Source: CAD feature listing. Evaluate the final solid. Frame: model axes, mm. A direction names the side the tool comes from. Round coordinates to 2 decimals unless told otherwise and drop trailing zeros. Loops run counter-clockwise (first coordinate to the right, second up) from the corner with the lowest first, then second, coordinate; pieces in that order, holes last.
Item 1: Section query C-C on y = 25. Return loops of the section in (x, z), then the cut area to 3 significant figures.
Item 2: Section query B-B on z = 16. Return loops of the section in (x, y), then the cut area to 3 significant figures.
Item 3: Section query D-D on z = 8. Return loops of the section in (x, y).
Item 4: Pull-direction query (Z, two-part tool) for faces 1 (the cylindrical face through (-47, 6.6, -6.5)), 2 (the flat face through (-1, 9, 28.5)), 3 (the flat face through (-1, 0, 0)), 4 (the cylindrical face through (-50.845, 6.591, 11.091)); classes: released by +Z, released by -Z, zero draft, split by the parting line, or undercut.
Item 5: Section query A-A on x = -44.5. Return loops of the section in (y, z), then the cut area to 3 significant figures.
Item 6: Access query for faces 5 (the flat face through (60.5, 9, 0)), 6 (the flat face through (46.811, 23.778, -10.444)), 7 (the flat face through (-25.5, 24, 0)), 8 (the flat face through (4, 35, 6.5)). Directions: +Z, -Z, +X, -X, +Y, -Y. A direction counts if a zero-diameter tool reaches every point of the face in a straight line with its end or side. Return the directions, or none.
Item 7: First-contact query: P1, Ø5, axis at x = -21.5, z = 5.5, coming from the +Y side; P2, Ø2, axis at x = 24.5, y = 25, coming from the +Z side; P3, Ø1.5, axis at x = -22, z = 11, coming from the +Y side; P4, Ø10.5, axis at x = -44.5, z = 12.5, coming from the -Y side (3 decimals). Flat tips, straight axial feed; report the tip coordinate or a pass-through.
Item 8: Ray query, L1, parallel to Z at x = -44, y = 10; L2, parallel to X at y = 2.5, z = -12.5; L3, parallel to Z at x = 3, y = 26. Return the intervals inside material, ascending.
```python
from build123d import *

# Parameters (mm, degrees)
SKETCH1_W           = 121
SKETCH1_H           = 57
BOSS_EXTRUDE1_DEPTH = 13
SKETCH3_W           = 86
SKETCH3_H           = 41
BOSS_EXTRUDE2_DEPTH = 57
CUT_EXTRUDE1_DEPTH  = 41
BOSS_EXTRUDE3_START = -57
BOSS_EXTRUDE3_DEPTH = 57
CUT_EXTRUDE3_DEPTH  = 100.122399083
CUT_EXTRUDE4_REACH  = 101.122
CUT_EXTRUDE5_REACH  = 101.122
SKETCH10_R          = 6.5
CUT_EXTRUDE6_DEPTH  = 79.444247718


with BuildPart() as part:
    # Sketch1 → Boss-Extrude1 (new body)
    with BuildSketch(Plane(origin=(0, 0, 0), x_dir=(1, 0, 0), z_dir=(0, 1, 0))):
        Rectangle(SKETCH1_W, SKETCH1_H)
    extrude(amount=BOSS_EXTRUDE1_DEPTH)

    # Sketch3 → Boss-Extrude2 (add)
    with BuildSketch(Plane.XY.offset(28.5)):
        with Locations((17.5, 33.5)):
            Rectangle(SKETCH3_W, SKETCH3_H)
    extrude(amount=-BOSS_EXTRUDE2_DEPTH)

    # Sketch5 → Cut-Extrude1 (cut)
    with BuildSketch(Plane(origin=(0, 54, 0), x_dir=(1, 0, 0), z_dir=(0, 1, 0))):
        Polygon((-25.5, -6.5), (33.5, -6.5), (60.5, -14.5), (60.5, -28.5), (-25.5, -28.5), align=None)
        Polygon((33.5, 6.5), (60.5, 14.5), (60.5, 28.5), (-25.5, 28.5), (-25.5, 6.5), align=None)
    extrude(amount=-CUT_EXTRUDE1_DEPTH, mode=Mode.SUBTRACT)

    # Sketch6 → Boss-Extrude3 (add)
    with BuildSketch(Plane.XY.offset(28.5).offset(BOSS_EXTRUDE3_START)):
        Polygon((-25.5, 32), (60.5, 8.956369451), (-25.5, 13), align=None)
    extrude(amount=BOSS_EXTRUDE3_DEPTH)

    # Sketch7 → Cut-Extrude3 (cut, through all)
    with BuildSketch(Plane.XY.offset(28.5)):
        Polygon((-25.5, 54), (33.536835762, 38.181127534), (60.5, 22.613937403), (60.5, 54), align=None)
    extrude(amount=-CUT_EXTRUDE3_DEPTH, mode=Mode.SUBTRACT)

    # Cut-Extrude4: up to this face of the body (flat: up to its plane)
    cut_extrude4_end = Plane(part.part.faces().sort_by_distance((45.301820021, 22.632080787, 9.996835562))[0])
    # Sketch8 → Cut-Extrude4 (cut, up to the picked face)
    with BuildSketch(Plane.XY.offset(28.5), mode=Mode.PRIVATE) as cut_extrude4_sk1:
        Polygon((45.408965344, 13), (60.5, 13), (60.5, 8.956369451), align=None)
    cut_extrude4_tool1 = split(extrude(cut_extrude4_sk1.sketch, amount=-CUT_EXTRUDE4_REACH, mode=Mode.PRIVATE), bisect_by=cut_extrude4_end, keep=Keep.BOTH, mode=Mode.PRIVATE)
    add(cut_extrude4_tool1.solids().sort_by(Axis((55.469655, 11.652123, 28.5), (0, 0, -1)))[0], mode=Mode.SUBTRACT)

    # Cut-Extrude5: up to this face of the body (flat: up to its plane)
    cut_extrude5_end = Plane(part.part.faces().sort_by_distance((45.301820021, 22.632080787, -9.996835562))[0])
    # Sketch9 → Cut-Extrude5 (cut, up to the picked face)
    with BuildSketch(Plane(origin=(0, 0, -28.5), x_dir=(-1, 0, 0), z_dir=(0, 0, -1)), mode=Mode.PRIVATE) as cut_extrude5_sk1:
        Polygon((-45.408965344, 13), (-60.5, 13), (-60.5, 8.956369451), align=None)
    cut_extrude5_tool1 = split(extrude(cut_extrude5_sk1.sketch, amount=-CUT_EXTRUDE5_REACH, mode=Mode.PRIVATE), bisect_by=cut_extrude5_end, keep=Keep.BOTH, mode=Mode.PRIVATE)
    add(cut_extrude5_tool1.solids().sort_by(Axis((55.469655, 11.652123, -28.5), (0, 0, 1)))[0], mode=Mode.SUBTRACT)

    # Sketch10 → Cut-Extrude6 (cut, through all)
    with BuildSketch(Plane(origin=(0, 13, 0), x_dir=(1, 0, 0), z_dir=(0, 1, 0))):
        with Locations(Location((-44.5, 12.5, 0), (0, 0, 270))):
            Circle(SKETCH10_R)
        with Locations(Location((-44.5, -12.5, 0), (0, 0, 270))):
            Circle(SKETCH10_R)
    extrude(amount=-CUT_EXTRUDE6_DEPTH, mode=Mode.SUBTRACT)


solid = part.part
```
Data:
1. outline: (-25.5, -28.5) - (0.62, -28.5) - (0.62, -6.5) - (33.5, -6.5) - (56.37, -13.28) - (56.37, 13.28) - (33.5, 6.5) - (0.62, 6.5) - (0.62, 28.5) - (-25.5, 28.5) - close
1. area: 2,370 mm2
2. outline: (-60.5, 0) - (-49.98, 0) - (-49.98, 13) - (-60.5, 13) - close; (-39.02, 0) - (60.5, 0) - (60.5, 8.96) - (-25.5, 32) - (-25.5, 13) - (-39.02, 13) - close
2. area: 2,070 mm2
3. outline: (-60.5, 0) - (-49.19, 0) - (-49.19, 13) - (-60.5, 13) - close; (-39.81, 0) - (60.5, 0) - (60.5, 22.61) - (38.56, 35.28) - (38.56, 14.83) - (-25.5, 32) - (-25.5, 13) - (-39.81, 13) - close
4. face 1: undercut
4. face 2: released by +Z
4. face 3: zero draft
4. face 4: undercut
5. outline: (0, -28.5) - (13, -28.5) - (13, -19) - (0, -19) - close; (0, -6) - (13, -6) - (13, 6) - (0, 6) - close; (0, 19) - (13, 19) - (13, 28.5) - (0, 28.5) - close
5. area: 403 mm2
6. face 5: +Z, -Z, +X, +Y, -Y
6. face 6: -Z, +Y
6. face 7: +Z, -Z, -X, +Y
6. face 8: +Z, +Y
7. P1: stops at y = 53.6
7. P2: stops at z = 6.5
7. P3: stops at y = 31.26
7. P4: passes through
8. L1: z = -28.5 to -18.98, -6.02 to 6.02, 18.98 to 28.5
8. L2: x = -60.5 to -51, -38 to 60.5
8. L3: z = -6.5 to 6.5
